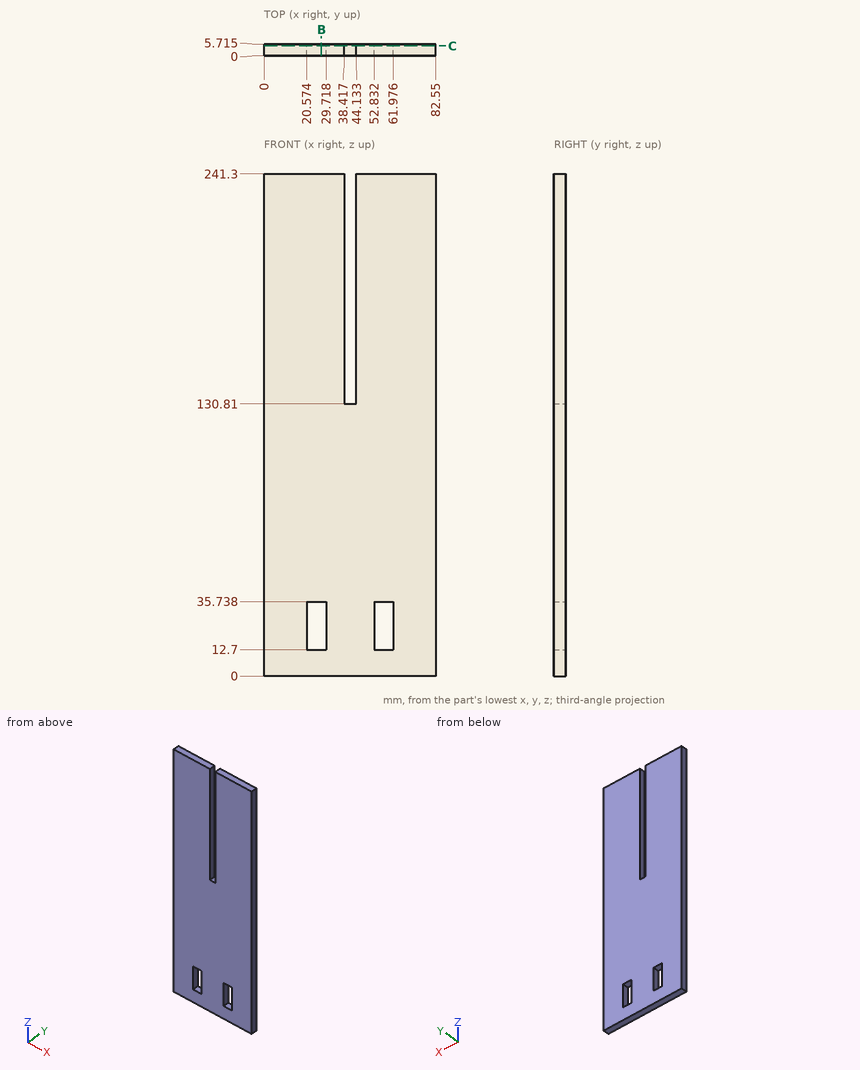
Source: three-view drawing plus pictorial views. Frame: mm from the lowest corner of the part. Give positions to 0.01 mm unless a question says otherwise; leave off trailing zeros. Write each loop counter-clockwise with the first axis right and the second up, starting at its lowest first coordinate (ties: lowest second). Pieces come first, ordered by that corner, then holes. Notation, with made-up numbers: (29, -10.75) - (70, -10.75) arc R18 ccw to (70, 3.25) - close; hole circle Ø6 at (85, 27). An arc over 180 degrees is marked (long way). Write item = value, one per line. Start each with the question number.
Q1. Cut plane C-C, the plane y = 4.85. Give the number of separate pieces and of enclosed holes in the cut face, then the cut area to 3 significant figures.
Q2. Material intervals for probe 1 along X at (y, z) = (1.4, 200); probe 2 along Z at (x, y) = (29.5, 5.3); probe 3 along Z at (x, y) = (42.5, 5.2), sorted ascending.
Q3. Pin query (flat end, axial travel): pin 1 Ø5 at (x, z) = (23, 68.5) entering from -Y. Return the tip coordinate at first contact, or that it passes through.
Q4. Cut plane B-B, the plane x = 27.5. Return loops of the section in (y, z) (1 decimal), then the cut area to 3 significant figures.
Computed values:
q1.separate_pieces = 1
q1.enclosed_holes = 2
q1.area = 18,900 mm²
q2.probe_1 = 0 to 38.42, 44.13 to 82.55
q2.probe_2 = 0 to 12.7, 35.74 to 241.3
q2.probe_3 = 0 to 130.81
q3.pin_1 = 0
q4.outline = (0, 0) - (5.7, 0) - (5.7, 12.7) - (0, 12.7) - close; (0, 35.7) - (5.7, 35.7) - (5.7, 241.3) - (0, 241.3) - close
q4.area = 1,250 mm²
